Verification items for the finished model (mm, model axes). A direction names the side the tool comes from. Round coordinates to 2 decimals unless told otherwise and drop trailing zeros. Write each loop counter-clockwise with the first axis right and the second up, starting at its lowest first coordinate (ties: lowest second). Pieces come first, ordered by that corner, then holes. Notation, with made-up numbers: (16.5, -35.5) -> (24.5, -35.5) arc R35 cw to (24.5, 3.5) -> close; hole circle Ø6 at (72.25, -31). An arc over 180 degrees is marked (long way). Use CSV: the item, a comma, the result in double quotes.
Autodesk Inventor part; units mm, degrees
ref_plane "YZ Plane" through (0, 0, 0) normal (1, 0, 0) x (0, 1, 0)
ref_plane "XZ Plane" through (0, 0, 0) normal (0, 1, 0) x (-1, 0, 0)
ref_plane "XY Plane" through (0, 0, 0) normal (0, 0, 1) x (1, 0, 0)
sketch "Sketch1" plane through (0, 0, 0) normal (0, 0, 1) x (1, 0, 0)
  line L0 (0, 0) -> (40.132, 0)
  line L1 (40.132, 0) -> (40.132, 48.26)
  line L2 (40.132, 48.26) -> (0, 48.26)
  line L3 (0, 48.26) -> (0, 0)
  line L4 (3.556, 44.704) -> (36.576, 44.704) construction
  line L5 (36.576, 44.704) -> (36.576, 1.524) construction
  line L6 (36.576, 1.524) -> (3.556, 1.524) construction
  line L7 (3.556, 1.524) -> (3.556, 44.704) construction
  line L8 (37.592, 1.016) -> (37.592, 45.72)
  line L9 (37.592, 45.72) -> (2.54, 45.72)
  line L10 (2.54, 45.72) -> (2.54, 1.016)
  line L11 (2.54, 1.016) -> (37.592, 1.016) construction
  line L12 (2.54, 1.016) -> (2.54, 0)
  line L13 (37.592, 1.016) -> (37.592, 0)
  line L14 (12.446, 25.654) -> (27.686, 25.654)
  point P0 (20.066, 48.26)
  point P1 (20.066, 44.704)
  point P2 (3.556, 23.114)
  point P3 (0, 24.13)
  point P4 (20.066, 25.654)
  dimension "d2" = 33.02
  dimension "d3" = 43.18
  dimension "d4" = 1.524
  dimension "d8" = 2.54
  dimension "d9" = 1.016
  dimension "d14" = 15.24
  dimension "d15" = 19.05
  dimension "d34" = 1.016
  dimension "d35" = 1.016
extrude "Extrusion1" add sketch "Sketch1" against normal blind 1.524
sketch "Sketch2" plane through (0, 0, 0) normal (0, 0, 1) x (1, 0, 0)
  line L0 (2.54, 1.016) -> (2.54, 0)
  line L1 (0, 48.26) -> (0, 0)
  line L2 (2.54, 45.72) -> (2.54, 1.016)
  line L3 (37.592, 45.72) -> (2.54, 45.72)
  line L4 (40.132, 48.26) -> (0, 48.26)
  line L5 (40.132, 0) -> (40.132, 48.26)
  line L6 (37.592, 1.016) -> (37.592, 0)
  line L7 (37.592, 1.016) -> (37.592, 45.72)
  line L8 (0, 0) -> (2.54, 0)
  line L9 (37.592, 0) -> (40.132, 0)
extrude "Extrusion2" add sketch "Sketch2" along normal blind 13.3856
sketch "Sketch3" plane through (0, 0, 0) normal (0, 0, 1) x (1, 0, 0)
  line L0 (2.54, 1.016) -> (37.592, 1.016)
  line L1 (2.54, 0) -> (37.592, 0)
  line L2 (2.54, 0) -> (2.54, 45.72)
  line L3 (37.592, 45.72) -> (37.592, 0)
  point P0 (0, 0)
extrude "Extrusion3" add sketch "Sketch3" along normal blind 4.775
sketch "Sketch4" plane through (0, 0, 0) normal (0, 0, 1) x (1, 0, 0)
  circle A0 centre (12.446, 25.654) radius 3.175
  circle A1 centre (27.686, 25.654) radius 3.175
  circle A2 centre (12.446, 25.654) radius 0.9652
  circle A3 centre (27.686, 25.654) radius 0.9652
  point P0 (0, 0)
  dimension "d16" = 6.35
  dimension "d18" = 1.9304
extrude "Extrusion4" add sketch "Sketch4" along normal blind 3.175
sketch "Sketch5" plane through (0, 0, 0) normal (0, 0, 1) x (1, 0, 0)
  circle A0 centre (12.446, 25.654) radius 3.175 construction
  circle A1 centre (27.686, 25.654) radius 3.175 construction
  line L0 (2.54, 1.016) -> (37.592, 1.016) construction
  line L1 (37.592, 1.016) -> (37.592, 45.72) construction
  line L2 (37.592, 45.72) -> (2.54, 45.72) construction
  line L3 (2.54, 45.72) -> (2.54, 1.016) construction
  line L4 (3.556, 44.704) -> (36.576, 44.704) construction
  line L5 (3.556, 1.524) -> (3.556, 44.704) construction
  line L6 (36.576, 44.704) -> (36.576, 1.524) construction
  line L7 (36.576, 1.524) -> (3.556, 1.524) construction
  line L8 (2.54, 1.016) -> (37.592, 1.016)
  line L9 (37.592, 1.016) -> (37.592, 3.048)
  line L10 (37.592, 3.048) -> (2.54, 3.048)
  line L11 (2.54, 3.048) -> (2.54, 1.016)
  line L12 (2.54, 45.72) -> (37.592, 45.72)
  line L13 (37.592, 45.72) -> (37.592, 43.18)
  line L14 (37.592, 43.18) -> (2.54, 43.18)
  line L15 (2.54, 43.18) -> (2.54, 45.72)
  point P0 (0, 0)
  dimension "d21" = 1.524
  dimension "d25" = 1.524
extrude "Extrusion5" add sketch "Sketch5" along normal blind 3.175
sketch "Sketch6" plane through (0, 0, 4.775) normal (0, 0, 1) x (1, 0, 0)
  line L0 (40.132, 0) -> (0, 0) construction
  line L1 (4.826, 0) -> (2.54, 0)
  line L2 (2.54, 0) -> (2.54, 1.016)
  line L3 (2.54, 1.016) -> (4.826, 1.016)
  line L4 (4.826, 1.016) -> (4.826, 0)
  line L5 (2.54, 0) -> (2.54, 45.72)
  line L6 (37.592, 1.016) -> (2.54, 1.016) construction
  line L7 (35.306, 0) -> (37.592, 0)
  line L8 (37.592, 0) -> (37.592, 1.016)
  line L9 (37.592, 1.016) -> (35.306, 1.016)
  line L10 (35.306, 1.016) -> (35.306, 0)
  dimension "d26" = 2.286
  dimension "d27" = 2.286
extrude "Extrusion6" add sketch "Sketch6" along normal up to surface (8.6106 mm away)
fillet "Fillet1" radius 2.286 2 edges at (37.592, 1.016, 8.2803) (2.54, 1.016, 8.2803)
chamfer "Chamfer2" distance 1.524 angle 45 2 edges at (9.271, 25.654, 0) (24.511, 25.654, 0)
fillet "Fillet2" radius 3.175 4 edges at (0, 0, 5.9308) (40.132, 0, 5.9308) (40.132, 48.26, 5.9308) (0, 48.26, 5.9308)
sketch "Sketch7" plane through (0, 0, -1.524) normal (0, 0, -1) x (-1, 0, 0)
  circle A0 centre (8.509, 24.13) radius 2.5527
  arc A1 (0, 45.085) -> (-3.175, 48.26) centre (-3.175, 45.085) ccw construction
  line L0 (-3.175, 48.26) -> (-36.957, 48.26) construction
  arc A2 (-36.957, 48.26) -> (-40.132, 45.085) centre (-36.957, 45.085) ccw construction
  line L1 (-40.132, 45.085) -> (-40.132, 3.175) construction
  arc A3 (-40.132, 3.175) -> (-36.957, 0) centre (-36.957, 3.175) ccw construction
  line L2 (-36.957, 0) -> (-3.175, 0) construction
  arc A4 (-3.175, 0) -> (0, 3.175) centre (-3.175, 3.175) ccw construction
  line L3 (0, 3.175) -> (0, 45.085) construction
  line L4 (-36.957, 48.26) -> (-3.175, 48.26) construction
  line L5 (-20.066, 48.26) -> (-20.066, 0) construction
  arc A5 (0, 36.83) -> (6.35, 30.48) centre (6.35, 36.83) ccw
  arc A6 (6.35, 17.78) -> (0, 11.43) centre (6.35, 11.43) ccw
  line L6 (6.35, 30.48) -> (8.509, 30.48)
  arc A7 (8.509, 17.78) -> (8.509, 30.48) centre (8.509, 24.13) ccw
  line L7 (8.509, 17.78) -> (6.35, 17.78)
  line L8 (0, 36.83) -> (0, 11.43)
  line L9 (0, 3.175) -> (0, 45.085)
  circle A8 centre (-48.641, 24.13) radius 2.5527
  arc A9 (-46.482, 30.48) -> (-40.132, 36.83) centre (-46.482, 36.83) ccw
  arc A10 (-40.132, 11.43) -> (-46.482, 17.78) centre (-46.482, 11.43) ccw
  line L10 (-46.482, 30.48) -> (-48.641, 30.48)
  arc A11 (-48.641, 30.48) -> (-48.641, 17.78) centre (-48.641, 24.13) ccw
  line L11 (-48.641, 17.78) -> (-46.482, 17.78)
  line L12 (-40.132, 36.83) -> (-40.132, 11.43)
  point P0 (0, 0)
  point P1 (0, 24.13)
  point P2 (-40.132, 24.13)
  dimension "d40" = 5.1054
  dimension "d41" = 6.35
  dimension "d43" = 6.35
  dimension "d44" = 57.15
extrude "Extrusion7" add sketch "Sketch7" against normal blind 5.08
fillet "Fillet3" radius 3.175 2 edges at (40.132, 24.13, 3.556) (0, 24.13, 3.556)
equation "\"d12\" = BoardOffset + PCBThickness"
equation "\"d19\" = BoardOffset"
equation "\"d23\" = BoardOffset"
equation "\"d27\" = d26"
equation "\"d28\" = BoardOffset"
equation "\"PCBThickness\" = 1.6"
equation "\"BoardOffset\" = 3.175"
properties part number "TOF Case P1"
Q1. Section check A-A (z = 12). Record the cut outline in (x, y) (3 decimals).
Filled in:
outline,"(0, 3.175) arc R3.175 ccw to (3.175, 0) -> (4.826, 0) -> (4.826, 1.016) arc R2.286 cw to (2.54, 3.302) -> (2.54, 45.72) -> (37.592, 45.72) -> (37.592, 3.302) arc R2.286 cw to (35.306, 1.016) -> (35.306, 0) -> (36.957, 0) arc R3.175 ccw to (40.132, 3.175) -> (40.132, 45.085) arc R3.175 ccw to (36.957, 48.26) -> (3.175, 48.26) arc R3.175 ccw to (0, 45.085) -> close"
Q2. Section check D-D (x = 44.5). Record the cut outline in (y, z), plus the area to 3 significant figures.
Filled in:
outline,"(17.46, -1.52) -> (30.8, -1.52) -> (30.8, 3.56) -> (17.46, 3.56) -> close"
area,"67.7 mm²"
Q3. Material ranges on L1, parallel to Y at x = 23, z = 1; L2, parallel to X at y = 9, z = 5.25; L3, parallel to Y at x = 4, z = 9.25, recorded low to high.
Filled in:
L1,"0 to 3.05, 43.18 to 48.26"
L2,"0 to 2.54, 37.59 to 40.13"
L3,"0 to 1.17, 45.72 to 48.26"
Q4. Mould release check, pull along X, two halves, no side actions. Record for faces 1 (the flat face through (20, 44, 3.175)), 2 (the cylindrical face through (42.04, 32.29, 1.63)), 3 (the flat face through (48, 30.48, 1)): released by +X, released by -X, zero draft, split by the parting line, or undercut.
Filled in:
face 1,"undercut"
face 2,"released by +X"
face 3,"zero draft"
Q5. Go/stop test with flat-tipped pins: P1, Ø1.1, axis at y = 0.5, z = 9.5, coming from the +X side; P2, Ø8, axis at y = 16, z = 9.5, coming from the -X side; P3, Ø3, axis at y = 43.5, z = 4.5, coming from the +X side. Record where each tip stops, or that it passes through.
Filled in:
P1,"x = 39.32"
P2,"x = -0.25"
P3,"x = 40.13"
Q6. Section check B-B (y = 14.5). Record the cut outline in (x, z) (3 decimals), plus the area to 3 significant figures.
Filled in:
outline,"(-0.791, -1.524) -> (40.923, -1.524) -> (40.923, 4.634) arc R3.175 cw to (40.132, 6.731) -> (40.132, 13.386) -> (37.592, 13.386) -> (37.592, 0) -> (2.54, 0) -> (2.54, 13.386) -> (0, 13.386) -> (0, 6.731) arc R3.175 cw to (-0.791, 4.634) -> close"
area,"140 mm²"
Q7. Section check C-C (x = -1.5). Record the cut outline in (y, z).
Filled in:
outline,"(15.53, -1.52) -> (32.73, -1.52) -> (32.73, 4.03) -> (15.53, 4.03) -> close"
Q8. Access from +Z, -Z, +X, -X, +Y, -Y to the whole of each face (thin tool, end or side, straight path). Record for faces 4 (the cylindrical face through (46.206, 24.897, 0.98)), 5 (the flat face through (48, 17.78, 1)), 6 (the flat face through (-6, 23, 3.556)), 7 (the flat face through (37.592, 24, 7)).
Filled in:
face 4,"+Z, -Z"
face 5,"+Z, -Z, +X, -Y"
face 6,"+Z, -X, +Y, -Y"
face 7,"+Z"
